Design review of the part shown in the three views and the two pictorial views. Dimensions are in mm from the part's minimum x, y and z. A direction names the side the tool comes from. Round coordinates to 2 decimals unless told otherwise and drop trailing zeros. Order: outer loops, then holes, each group sorted by start corner. A loop starts at its lowest first (then second) coordinate and runs counter-clockwise, first axis right, second up.
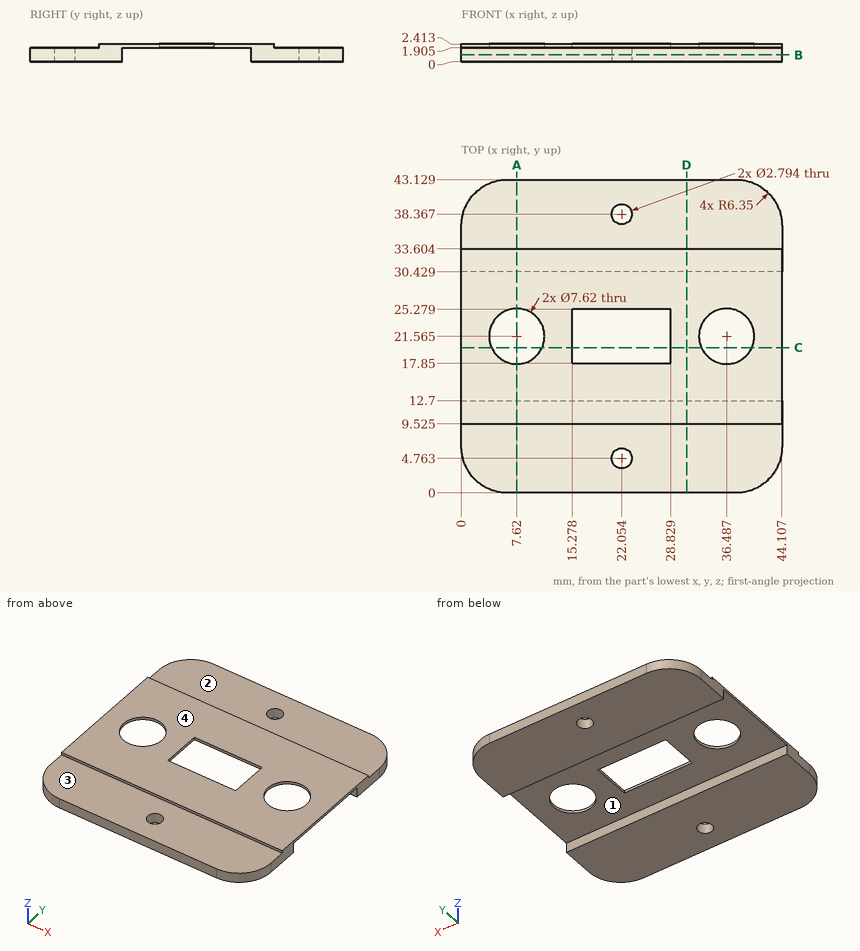
(1) Draft analysis for pull direction Y (two halves, no side actions). For the marked faces 1 and 2, state which applies: pulls with the +Y half, pulls with the -Y half, needs draft (parallel to the pull), parting line crosses it, or undercut.
Data:
face 1: undercut
face 2: needs draft
(2) For the marked faces 3 and 4, list the 3-axis set-ups (+Z, -Z, +X, -X, +Y, -Y) from which the entire face can be reached by the end or side of a thin tool; tool diameter is ignored.
Data:
face 3: +Z, +X, -X, -Y
face 4: +Z, +X, -X, +Y, -Y
(3) Consider section D-D (x = 31). Write out the cut boundary in (y, z) (1 decimal).
Data:
outline: (0, 0) - (12.7, 0) - (12.7, 1.9) - (30.4, 1.9) - (30.4, 0) - (43.1, 0) - (43.1, 1.9) - (33.6, 1.9) - (33.6, 2.4) - (9.5, 2.4) - (9.5, 1.9) - (0, 1.9) - close
(4) Consider section A-A (x = 7.62). Write out the cut boundary in (y, z) (1 decimal).
Data:
outline: (0, 0) - (12.7, 0) - (12.7, 1.9) - (17.8, 1.9) - (17.8, 2.4) - (9.5, 2.4) - (9.5, 1.9) - (0, 1.9) - close; (25.4, 1.9) - (30.4, 1.9) - (30.4, 0) - (43.1, 0) - (43.1, 1.9) - (33.6, 1.9) - (33.6, 2.4) - (25.4, 2.4) - close
(5) Insertion check: pin 1 (7.5 mm diameter, centred on x = 20, y = 40, fed in from +Z) (1 decimal); pin 2 (4 mm diameter, centred on x = 10, y = 22.5, fed in from -Z) (1 decimal); pin 3 (2 mm diameter, centred on x = 22.05, y = 4.76, fed in from +Z). Each pin has a flat end and moves straight along its axis. Give the tip position at first contact, or say it passes through.
Data:
pin 1: stops at z = 1.9
pin 2: stops at z = 1.9
pin 3: passes through
(6) Consider section B-B (z = 0.9). State how many separate pieces and enclosed holes the cut face has, and give its area (3 significant figures).
Data:
separate pieces: 2
enclosed holes: 2
area: 1,070 mm2
(7) To check wall thickness, follow probe 1 along Y at (x, z) = (12, 0.4); probe 2 along Z at (x, y) = (8.5, 15) (1 decimal); probe 3 along Z at (x, y) = (12, 41.5) (1 decimal). State the ranges of each line that lie inside material, in increasing order.
Data:
probe 1: y = 0 to 12.7, 30.43 to 43.13
probe 2: z = 1.9 to 2.4
probe 3: z = 0 to 1.9
(8) Consider section C-C (y = 20). Write out the cut boundary in (x, z) (1 decimal).
Data:
outline: (0, 1.9) - (4.1, 1.9) - (4.1, 2.4) - (0, 2.4) - close; (11.1, 1.9) - (15.3, 1.9) - (15.3, 2.4) - (11.1, 2.4) - close; (28.8, 1.9) - (33, 1.9) - (33, 2.4) - (28.8, 2.4) - close; (40, 1.9) - (44.1, 1.9) - (44.1, 2.4) - (40, 2.4) - close
